For this review, take the finished solid that the model builds, in its own axes (mm). A direction names the side the tool comes from. Give positions to 0.01 mm unless a question says otherwise; leave off trailing zeros. Write each loop counter-clockwise with the first axis right and the second up, starting at its lowest first coordinate (ties: lowest second). Pieces come first, ordered by that corner, then holes.
Q1. Insertion check: P1, Ø5, axis at x = 57, z = -204, coming from the +Y side; P2, Ø9, axis at x = 446, y = 130.5, coming from the +Z side; P3, Ø5, axis at x = 136.5, y = 19, coming from the -Z side; P4, Ø9, axis at x = 444, y = 139, coming from the -Z side. Each pin has a flat end and moves straight along its axis. Give the tip position at first contact, or say it passes through.
Q2. Machinability: for faces 5 (the flat face through (222, 0, -152)), 6 (the flat face through (451, 68, -115)), 7 (the flat face through (18, 81, -115)), 8 (the flat face through (442, 150.25, -81)), 9 (the flat face through (442, 101.06, -213)), which of the approach directions +Z, -Z, +X, -X, +Y, -Y give a long, thin tool a straight path to every point of the face, cutting with its end or side? Answer none if there is none.
Q3. We need section C-C (z = -228.5). Write out the cut boundary in (x, y).
Q4. We need section A-A (z = -81.5). Write out the cut boundary in (x, y), then the cut area to 3 significant figures.
Q5. For line 1 (X direction, y = 30, z = -184); line 2 (Y direction, x = 8.75, z = -81.5); line 3 (Y direction, x = 12.5, z = -206.89), list the stretches that pass through material, from the lowest coordinate up.
Q6. Mouldability with a two-part tool opening along Z and no side actions: class faces 1 (the flat face through (442, 178.261, -81)), 2 (the flat face through (442, 107.75, -81)), 3 (the flat face through (442, 129, -60.25)), 4 (the flat face through (8.87, 70.16, -282.35)) as released by +Z, released by -Z, zero draft, split by the parting line, or undercut.
Q7. We need section B-B (y = 90.5). Write out the cut boundary in (x, z), then the cut area to 3 significant figures.
Q8. We need section D-D (y = 129). Write out the cut boundary in (x, z), then the cut area to 3 significant figures.
```python
from build123d import *

# Parameters (mm, degrees)
SKETCH1_W           = 451
SKETCH1_H           = 300
BOSS_EXTRUDE6_DEPTH = 18
SKETCH4_R           = 4
SKETCH4_W           = 42.5
SKETCH4_H           = 42.5
BOSS_EXTRUDE7_DEPTH = 18
SKETCH5_R           = 10.85
SKETCH5_R_2         = 4
BOSS_EXTRUDE8_DEPTH = 18


with BuildPart() as part:
    # Sketch1 → Boss-Extrude6 (new body)
    with BuildSketch(Plane(origin=(0, 0, 0), x_dir=(1, 0, 0), z_dir=(0, 1, 0))):
        with Locations((225.5, 150)):
            Rectangle(SKETCH1_W, SKETCH1_H)
    extrude(amount=BOSS_EXTRUDE6_DEPTH)

    # Sketch4 → Boss-Extrude7 (add)
    with BuildSketch(Plane(origin=(451, 0, 0), x_dir=(0, 0, -1), z_dir=(1, 0, 0))):
        Polygon((0, 0), (0, 101.059625538), (45.34233012, 178.261418028), (117.954980558, 178.261418028), (163.295274024, 101.059625538), (264.202994821, 101.059625538), (300, 40.107374144), (300, 0), align=None)
        with Locations((206.89, 66.5)):
            Circle(SKETCH4_R, mode=Mode.SUBTRACT)
        with Locations((270.64, 66.5)):
            Circle(SKETCH4_R, mode=Mode.SUBTRACT)
        with Locations((81.5, 129)):
            Rectangle(SKETCH4_W, SKETCH4_H, mode=Mode.SUBTRACT)
    extrude(amount=-BOSS_EXTRUDE7_DEPTH)

    # Sketch5 → Boss-Extrude8 (add)
    with BuildSketch(Plane.ZY):
        Polygon((-300, 0), (-300, 40.107374144), (-264.202994821, 101.059625538), (-163.295274024, 101.059625538), (-117.954980558, 178.261418028), (-45.34233012, 178.261418028), (0, 101.059625538), (0, 0), align=None)
        with Locations((-81.5, 129)):
            Circle(SKETCH5_R, mode=Mode.SUBTRACT)
        with Locations((-270.64, 66.5)):
            Circle(SKETCH5_R_2, mode=Mode.SUBTRACT)
        with Locations((-206.89, 66.5)):
            Circle(SKETCH5_R_2, mode=Mode.SUBTRACT)
    extrude(amount=-BOSS_EXTRUDE8_DEPTH)


solid = part.part
```
Computed:
1. P1: stops at y = 18
1. P2: stops at z = -14.65
1. P3: stops at z = -300
1. P4: stops at z = -143.66
2. face 5: +Z, -Z, +X, -X, -Y
2. face 6: +Z, -Z, +X, +Y, -Y
2. face 7: +Z, -Z, +Y
2. face 8: +X
2. face 9: -Z, +X, -X, +Y
3. outline: (0, 0) - (451, 0) - (451, 101.06) - (433, 101.06) - (433, 18) - (18, 18) - (18, 101.06) - (0, 101.06) - close
4. outline: (0, 0) - (451, 0) - (451, 107.75) - (433, 107.75) - (433, 18) - (18, 18) - (18, 118.15) - (0, 118.15) - close; (0, 139.85) - (18, 139.85) - (18, 178.26) - (0, 178.26) - close; (433, 150.25) - (451, 150.25) - (451, 178.26) - (433, 178.26) - close
4. area: 12,700 mm2
5. line 1: x = 0 to 18, 433 to 451
5. line 2: y = 0 to 118.15, 139.85 to 178.26
5. line 3: y = 0 to 62.5, 70.5 to 101.06
6. face 1: zero draft
6. face 2: undercut
6. face 3: undercut
6. face 4: released by -Z
7. outline: (0, -270.4) - (18, -270.4) - (18, 0) - (0, 0) - close; (433, -270.4) - (451, -270.4) - (451, 0) - (433, 0) - close
7. area: 9,730 mm2
8. outline: (0, -146.89) - (18, -146.89) - (18, -92.35) - (0, -92.35) - close; (0, -70.65) - (18, -70.65) - (18, -16.41) - (0, -16.41) - close; (433, -146.89) - (451, -146.89) - (451, -102.75) - (433, -102.75) - close; (433, -60.25) - (451, -60.25) - (451, -16.41) - (433, -16.41) - close
8. area: 3,540 mm2
